Read the model definition and answer for the solid it produces. Units are mm, in the model's axes. Round coordinates to 2 decimals unless told otherwise and drop trailing zeros. Loops run counter-clockwise (first coordinate to the right, second up) from the corner with the lowest first, then second, coordinate; pieces in that order, holes last. Notation, with made-up numbers: M 37,25 L 71,25 A25 ccw 71,48 Z; hole C -14.75,77 d5. An arc over 180 degrees is marked long. Write each question's results on one line, items separated by ' | '.
```python
from build123d import *

# Parameters (mm, degrees)
F1_DEPTH = 10


# Not quite as in the source:
# - the program builds the solid bodies; features that only make, move or delete a surface that nothing else refers to are left out


with BuildPart() as f1:
    # F0 (on Front) → F1 (new body)
    with BuildSketch(Plane.XZ):
        with BuildLine():
            ThreePointArc((-8.1000001146, 0), (-13.3357647385, 15.3093108924), (-26.8500001146, 24.2061459138))
            ThreePointArc((-26.8500001146, 24.2061459138), (-58.1000001146, 0), (-26.8500001146, -24.2061459138))
            ThreePointArc((-26.8500001146, -24.2061459138), (-13.3357647385, -15.3093108924), (-8.1000001146, 0))
        make_face()
        with BuildLine():
            Line((20.0249998854, 12.1030729569), (-26.8500001146, 24.2061459138))
            ThreePointArc((-26.8500001146, 24.2061459138), (-13.3357647385, 15.3093108924), (-8.1000001146, 0))
            ThreePointArc((-8.1000001146, 0), (-13.3357647385, -15.3093108924), (-26.8500001146, -24.2061459138))
            Line((-26.8500001146, -24.2061459138), (20.0249998854, -12.1030729569))
            ThreePointArc((20.0249998854, -12.1030729569), (4.3999998854, 0), (20.0249998854, 12.1030729569))
        make_face()
        with BuildLine():
            ThreePointArc((29.3999998854, 0), (26.7821175735, 7.6546554462), (20.0249998854, 12.1030729569))
            ThreePointArc((20.0249998854, 12.1030729569), (4.3999998854, 0), (20.0249998854, -12.1030729569))
            ThreePointArc((20.0249998854, -12.1030729569), (26.7821175735, -7.6546554462), (29.3999998854, 0))
        make_face()
    extrude(amount=F1_DEPTH)


solid = f1.part
```
1. Find the intervals of material crossed by L1, parallel to Z at x = -37.5, y = -1; L2, parallel to Z at x = -42, y = -6.5; L3, parallel to X at y = -4.75, z = -1, in increasing order.
Completed:
L1: z = -24.61 to 24.61 | L2: z = -23.36 to 23.36 | L3: x = -58.08 to 29.36
2. Given P1, Ø5, axis at x = -18.5, y = -1.5, coming from the +Z side; P2, Ø2, axis at x = -14, y = -2, coming from the +Z side; P3, Ø6, axis at x = -27.5, y = -5.5, coming from the -Z side, each flat-ended and moving along its own axis, determine where each tip first touches the part or whether it passes through.
Completed:
P1: stops at z = 22.7 | P2: stops at z = 21.15 | P3: stops at z = -24.86
3. Find section B-B, the plane z = 14.5. Give the vertices of the cut face in (x, y), then the cut area to 3 significant figures.
Completed:
outline: M -53.47,-10 L 10.74,-10 L 10.74,0 L -53.47,0 Z | area: 642 mm2
4. Find section C-C, the plane x = 4.5. Give the vertices of the cut face in (y, z).
Completed:
outline: M -10,-16.11 L 0,-16.11 L 0,16.11 L -10,16.11 Z
5. Find section A-A, the plane y = -7.5. Give the vertices of the cut face in (x, z) (3 decimals), then the cut area to 3 significant figures.
Completed:
outline: M -26.85,-24.206 L 20.025,-12.103 A12.5 ccw 20.025,12.103 L -26.85,24.206 A25 ccw long Z | area: 3,160 mm2
